Geometry check sheet. Reference: drawing and pictorial views, mm from the part's lowest x, y, z. Give positions to 0.01 mm unless a question says otherwise; leave off trailing zeros. Loops run counter-clockwise (first coordinate to the right, second up) from the corner with the lowest first, then second, coordinate; pieces in that order, holes last. Notation, with made-up numbers: (52.25, 23) -> (69.25, 23) arc R21 cw to (69.25, 55) -> close; hole circle Ø9 at (84.5, 12.25). An arc over 180 degrees is marked (long way). Write each question's results on one line, items separated by ' | '. Start each with the question number.
1. Material ranges on L1, parallel to Y at x = 4, z = 22; L2, parallel to X at y = 4.25, z = 45; L3, parallel to Y at x = 4.5, z = 8, recorded low to high. Write a range as from..to.
2. Cross-section at B-B on z = 27.5. Record the boundary of the cut face in (x, y), and give its area (3 significant figures).
3. Mould release check, pull along Y, two halves, no side actions. Record for the marked faces 1, 2 and 3: +Y half, -Y half, draft (parallel to the pull), parting line (faces both ways), or undercut.
4. Gauge pin test, flat ends, axial feed: pin 1 Ø1.5 at (y, z) = (6, 21.5) entering from +X; pin 2 Ø2 at (x, y) = (2.5, 4) entering from -Z; pin 3 Ø3 at (y, z) = (7, 12.5) entering from -X; pin 4 Ø1.5 at (x, y) = (6.5, 6.5) entering from +Z. Record the tip position at first contact, or that the pin passes through.
5. Cross-section at A-A on z = 40.5. Record the boundary of the cut face in (x, y).
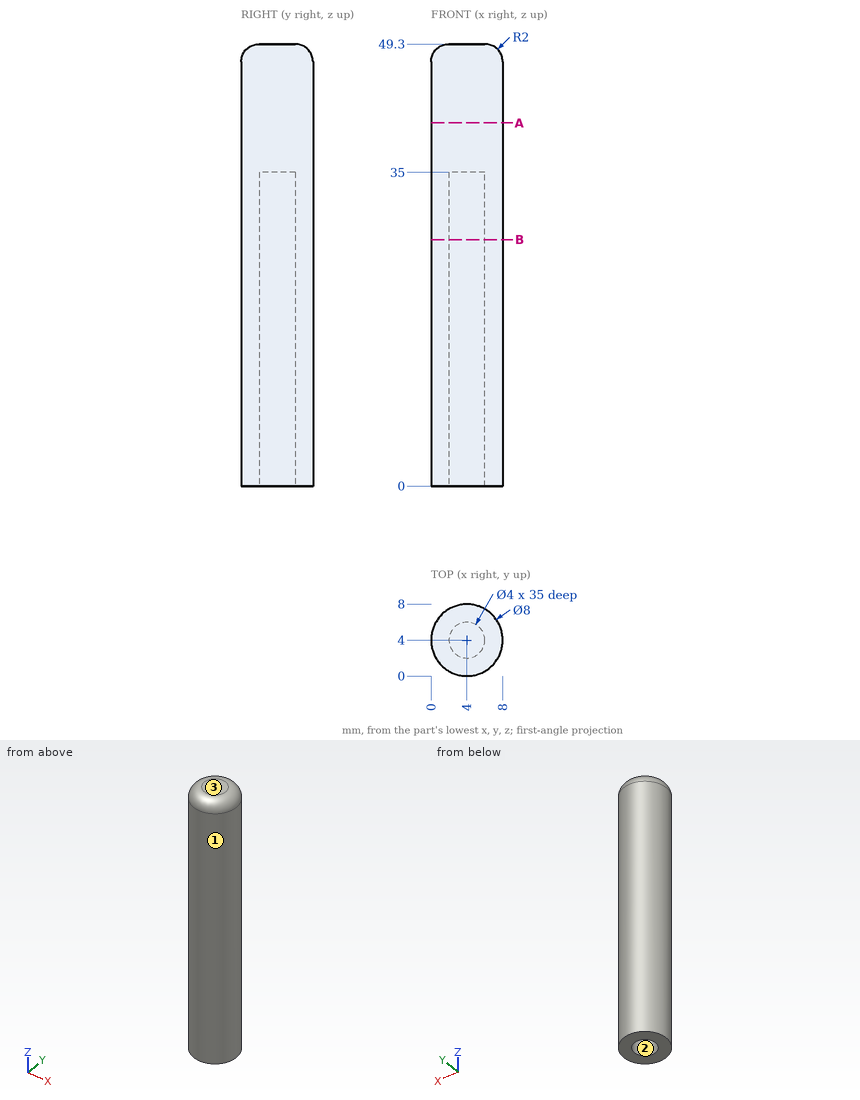
Geometry says:
1) L1: 0..2, 6..8 | L2: 0.01..7.99 | L3: 0.03..2.06, 5.94..7.97
2) outline: circle Ø8 at (4, 4); hole circle Ø4 at (4, 4) | area: 37.7 mm^2
3) face 1: parting line | face 2: undercut | face 3: draft
4) pin 1: x = 7.8 | pin 2: z = 0 | pin 3: x = 0.29 | pin 4: z = 49.14
5) outline: circle Ø8 at (4, 4)
